```python
from build123d import *


with BuildPart() as part:
    # Эскиз1 → Повернуть1 (revolve)
    with BuildSketch(Plane(origin=(0, 0, 0), x_dir=(0, 0, -1), z_dir=(1, 0, 0)), mode=Mode.PRIVATE) as revolve_1_sk:
        with BuildLine():
            Line((-39.358214094, 0), (-39.358214094, 2))
            Line((-39.358214094, 2), (-38.358214094, 3))
            Line((-38.358214094, 3), (-7.358214094, 3.62))
            Line((-7.358214094, 3.62), (-7.358214094, 3))
            Line((-7.358214094, 3), (8.641785906, 3))
            Line((8.641785906, 3), (8.641785906, 2))
            Line((8.641785906, 2), (9.641785906, 2))
            add(Edge.make_bspline(
                [(9.641785906, 2), (10.641785906, 1), (10.641785906, 0)],
                knots=[0, 0, 0, 0.5, 0.5, 0.5], degree=2))
            Line((10.641785906, 0), (-39.358214094, 0))
        make_face()
    revolve(revolve_1_sk.sketch.rotate(Axis((0, 0, 39.358214094), (0, 0, -1)), 90), axis=Axis((0, 0, 39.358214094), (0, 0, -1)))


solid = part.part
```
The model under review builds one solid part; all positions refer to its coordinate system, in mm. A direction names the side the tool comes from. Give positions to 0.01 mm unless a question says otherwise; leave off trailing zeros. Write each loop counter-clockwise with the first axis right and the second up, starting at its lowest first coordinate (ties: lowest second). Pieces come first, ordered by that corner, then holes. Notation, with made-up numbers: M 70.5,12.5 L 111.5,12.5 A13 cw 111.5,34.5 Z; hole C -26,11.5 d4. An arc over 180 degrees is marked long. Write item = value, one per line. Start each with the question number.
Q1. We need section A-A (z = 0). State the section outline as (x, y) points.
Q2. For line 1 (X direction, y = -0.25, z = 0); line 2 (Y direction, x = -1.5, z = 10); line 3 (Z direction, x = 1.5, y = -1.5), list the stretches that pass through material, from the lowest coordinate up.
Q3. We need section B-B (z = 17). State the section outline as (x, y) points, plus the area to 3 significant figures.
Q4. Clearance check with flat-ended pins moving along their axes: pin 1 (1 mm diameter, centred on x = 2.5, z = 13.5, fed in from -Y); pin 2 (1.8 mm diameter, centred on x = 1.5, y = -0.5, fed in from -Z); pin 3 (1.5 mm diameter, centred on x = 1.5, y = 1, fed in from -Z). State where each tip first meets the part, or that it passes through.
Q5. Machinability: for faces 1 (the face through (1, 2, -8.642)), 2 (the face through (0, 0, 39.358)), 3 (the face through (-0.718, 3.236, 22.641)), which of the approach directions +Z, -Z, +X, -X, +Y, -Y give a long, thin tool a straight path to every point of the face, cutting with its end or side? Answer none if there is none.
Result set:
q1.outline = C 0,0 d6
q2.line_1 = -2.99 to 2.99
q2.line_2 = -3.24 to 3.24
q2.line_3 = -8.64 to 39.24
q3.outline = C 0,0 d6.85
q3.area = 36.9 mm2
q4.pin_1 = -2.87
q4.pin_2 = -10.53
q4.pin_3 = -10.36
q5.face_1 = -Z
q5.face_2 = +Z, +X, -X, +Y, -Y
q5.face_3 = +Z
